```python
from build123d import *

# Parameters (mm, degrees)
SKETCH1_W           = 100
SKETCH1_H           = 100
BOSS_EXTRUDE1_DEPTH = 4
SKETCH2_W           = 100
SKETCH2_H           = 100
SKETCH2_W_2         = 92
SKETCH2_H_2         = 92
BOSS_EXTRUDE2_DEPTH = 35
SKETCH3_W           = 4
SKETCH3_H           = 4
CUT_EXTRUDE1_DEPTH  = 4
BOSS_EXTRUDE3_DEPTH = 2.5
SKETCH5_W           = 5.75
SKETCH5_H           = 4
CUT_EXTRUDE2_DEPTH  = 4


with BuildPart() as part:
    # Sketch1 → Boss-Extrude1 (new body)
    with BuildSketch(Plane(origin=(0, 0, 0), x_dir=(1, 0, 0), z_dir=(0, 1, 0))):
        Rectangle(SKETCH1_W, SKETCH1_H)
    extrude(amount=BOSS_EXTRUDE1_DEPTH)

    # Sketch2 → Boss-Extrude2 (add)
    with BuildSketch(Plane(origin=(0, 4, 0), x_dir=(1, 0, 0), z_dir=(0, 1, 0))):
        Rectangle(SKETCH2_W, SKETCH2_H)
        Rectangle(SKETCH2_W_2, SKETCH2_H_2, mode=Mode.SUBTRACT)
    extrude(amount=BOSS_EXTRUDE2_DEPTH)

    # Sketch3 → Cut-Extrude1 (cut)
    with BuildSketch(Plane(origin=(0, 0, -50), x_dir=(-1, 0, 0), z_dir=(0, 0, -1))):
        with Locations((0, 37)):
            Rectangle(SKETCH3_W, SKETCH3_H)
    extrude(amount=-CUT_EXTRUDE1_DEPTH, mode=Mode.SUBTRACT)

    # Sketch4 → Boss-Extrude3 (add)
    with BuildSketch(Plane(origin=(0, 4, 0), x_dir=(1, 0, 0), z_dir=(0, 1, 0))):
        Polygon((-1.75, -0.5), (0.75, -0.5), (0.75, 2), (-4.25, 2), (-4.25, -3), (-1.75, -3), align=None)
        Polygon((7.25, -0.5), (9.75, -0.5), (9.75, -3), (12.25, -3), (12.25, 2), (7.25, 2), align=None)
        Polygon((12.25, -14.5), (9.75, -14.5), (9.75, -17), (7.25, -17), (7.25, -19.5), (12.25, -19.5), align=None)
        Polygon((-1.75, -17), (-1.75, -14.5), (-4.25, -14.5), (-4.25, -19.5), (0.75, -19.5), (0.75, -17), align=None)
    extrude(amount=BOSS_EXTRUDE3_DEPTH)

    # Sketch5 → Cut-Extrude2 (cut)
    with BuildSketch(Plane(origin=(0, 4, 0), x_dir=(1, 0, 0), z_dir=(0, 1, 0))):
        with Locations((1.125, -15)):
            Rectangle(SKETCH5_W, SKETCH5_H)
    extrude(amount=-CUT_EXTRUDE2_DEPTH, mode=Mode.SUBTRACT)


solid = part.part
```
CAD build for the part. Positions are in the model's coordinates, mm. A direction names the side the tool comes from. Round coordinates to 2 decimals unless told otherwise and drop trailing zeros. Loops run counter-clockwise (first coordinate to the right, second up) from the corner with the lowest first, then second, coordinate; pieces in that order, holes last. Notation, with made-up numbers: (62.25, 13) - (118.25, 13) arc R11 ccw to (118.25, 23) - close; hole circle Ø9 at (-10.5, -38.5). An arc over 180 degrees is marked (long way). Return JSON: item names as keys, results as strings. Group by question number.
Q1. Drill centre lines: line 1 along Z through (x, y) = (17.5, 17); line 2 along Y through (x, z) = (6.5, 25). Where is each one in solid material? Low to high. Write a range as [from, to].
Q2. Two-plate mould, pull along X, no slides. Class faces 4 (the face through (50, 19, 1)), 5 (the face through (-4, 39, -48)), 6 (the face through (10, 5, 19.5)): +X half, -X half, draft (parallel to the pull), parting line (faces both ways), or undercut.
Q3. Flat gauge pin, fed straight in: pin 1 Ø4 at (x, z) = (9.5, 1) entering from +Y. Where does the tip first touch, or does it go through?
Q4. Band-saw the part on A-A on y = 18. Give the cut face in (x, z), plus the area to 3 significant figures.
Q5. Band-saw the part on C-C on z = 32. Give the cut face in (x, y).
Q6. Tool access for faces 1 (the face through (4, 2, 15)), 2 (the face through (-2, 6.5, 0)), 3 (the face through (-1, 19, 50)): list every direction of +Z, -Z, +X, -X, +Y, -Y with a clear straight run to the whole face (end or side of a thin tool).
Q7. Band-saw the part on B-B on x = -20. Give the cut face in (y, z).
Solutions:
{
 "1": {"line 1": "z = [-50, -46], [46, 50]", "line 2": "y = [0, 4]"},
 "2": {"face 4": "+X half", "face 5": "draft", "face 6": "undercut"},
 "3": {"pin 1": "stops at y = 6.5"},
 "4": {"outline": "(-50, -50) - (50, -50) - (50, 50) - (-50, 50) - close; hole (-46, -46) - (46, -46) - (46, 46) - (-46, 46) - close", "area": "1,540 mm^2"},
 "5": {"outline": "(-50, 0) - (50, 0) - (50, 39) - (46, 39) - (46, 4) - (-46, 4) - (-46, 39) - (-50, 39) - close"},
 "6": {"face 1": "+Y, -Y", "face 2": "+Y", "face 3": "+Z, +X, -X, +Y, -Y"},
 "7": {"outline": "(0, -50) - (39, -50) - (39, -46) - (4, -46) - (4, 46) - (39, 46) - (39, 50) - (0, 50) - close"}
}
